Source: CAD feature listing. Evaluate the final solid. Frame: model axes, mm. A direction names the side the tool comes from. Round coordinates to 2 decimals unless told otherwise and drop trailing zeros. Loops run counter-clockwise (first coordinate to the right, second up) from the corner with the lowest first, then second, coordinate; pieces in that order, holes last. Notation, with made-up numbers: M -22,73 L -5,73 A26 cw -5,108 Z; hole C 1.5,-6 d11. An arc over 180 degrees is marked long. Write each question's results on one line, items separated by ' | '. Start each with the question number.
1. Section A-A on y = 47. Output: boundary loops of the cut face in (x, z), and give its area (3 significant figures).
2. Ray query, line 1 (Y direction, x = 1.3, z = 9); line 2 (X direction, y = 2.55, z = 59); line 3 (Y direction, x = 1.65, z = 64.25). Return the intervals inside material, ascending.
3. Set-up query: faces 1 (the flat face through (22, 4, 34)), 2 (the cylindrical face through (2.028, 20.808, 62.022)). Return all of +Z, -Z, +X, -X, +Y, -Y with unobstructed straight access to the full face (end or side cutting, diameter ignored); none if empty.
4. Section B-B on z = 9. Output: boundary loops of the cut face in (x, y).
5. Section D-D on y = 14. Output: boundary loops of the cut face in (x, z).
6. Section C-C on x = 11.5. Output: boundary loops of the cut face in (y, z), and give its area (3 significant figures).
7. Draft query along Y for faces 3 (the cylindrical face through (1.97, 50.07, 62.55)), 4 (the cylindrical face through (11.773, 1.972, 6.918)), 5 (the flat face through (2, 54, 34)). Return one class per face: released by +Y, released by -Y, zero draft, split by the parting line, or undercut.
8. Contact query for flat-ended pins moving along their axis: pin 1 Ø5 at (x, z) = (11.5, 9) entering from -Y; pin 2 Ø5.5 at (y, z) = (14, 3.75) entering from +X; pin 3 Ø1.2 at (y, z) = (20.5, 63) entering from +X; pin 4 Ø5 at (x, z) = (33, 27) entering from +Y. Output: stop coordinate, or through.
from build123d import *

# Parameters (mm, degrees)
BOSS_EXTRUDE1_DEPTH          = 68
M3_CLEARANCE_HOLE1_D         = 3.4
M3_CLEARANCE_HOLE1_DEPTH     = 5
M3_CLEARANCE_HOLE1_TIP       = 1.021463052
M5X0_8_TAPPED_HOLE1_D        = 4.2
M5X0_8_TAPPED_HOLE1_DEPTH    = 14
M5X0_8_TAPPED_HOLE1_TIP      = 1.2618073
FILLET1_R                    = 4
CHAMFER1_SIZE                = 0.5
M2_5X0_45_TAPPED_HOLE1_D     = 2.05
M2_5X0_45_TAPPED_HOLE1_DEPTH = 7.25
M2_5X0_45_TAPPED_HOLE1_TIP   = 0.615882135
M3X0_5_TAPPED_HOLE3_D        = 2.5
M3X0_5_TAPPED_HOLE3_DEPTH    = 8.5
M3X0_5_TAPPED_HOLE3_TIP      = 0.751075774


with BuildPart() as part:
    # Sketch1 → Boss-Extrude1 (new body)
    with BuildSketch(Plane.XY):
        Polygon((0, 0), (39, 0), (39, 4), (4, 4), (4, 54), (0, 54), align=None)
    extrude(amount=BOSS_EXTRUDE1_DEPTH)

    # M3 Clearance Hole1
    with Locations(Plane(origin=(4, 0, 0), x_dir=(0, 0, -1), z_dir=(1, 0, 0))):
        with Locations((-64.25, 50), (-3.75, 50), (-3.75, 14), (-64.25, 14)):
            Hole(M3_CLEARANCE_HOLE1_D / 2, depth=M3_CLEARANCE_HOLE1_DEPTH)
            with Locations((0, 0, -(M3_CLEARANCE_HOLE1_DEPTH + M3_CLEARANCE_HOLE1_TIP / 2))):  # 118° drill point
                Cone(0, M3_CLEARANCE_HOLE1_D / 2, M3_CLEARANCE_HOLE1_TIP, mode=Mode.SUBTRACT)

    # M5x0.8 Tapped Hole1
    with Locations(Plane(origin=(0, 4, 0), x_dir=(1, 0, 0), z_dir=(0, 1, 0))):
        with Locations((31.5, -59), (11.5, -59), (11.5, -9), (31.5, -9)):
            Hole(M5X0_8_TAPPED_HOLE1_D / 2, depth=M5X0_8_TAPPED_HOLE1_DEPTH)
            with Locations((0, 0, -(M5X0_8_TAPPED_HOLE1_DEPTH + M5X0_8_TAPPED_HOLE1_TIP / 2))):  # 118° drill point
                Cone(0, M5X0_8_TAPPED_HOLE1_D / 2, M5X0_8_TAPPED_HOLE1_TIP, mode=Mode.SUBTRACT)

    # Fillet1
    fillet1_edges = [part.edges().sort_by_distance(p)[0] for p in [
        (2, 54, 68),
        (2, 54, 0),
    ]]
    fillet(fillet1_edges, radius=FILLET1_R)

    # Chamfer1
    chamfer1_edges = [part.edges().sort_by_distance(p)[0] for p in [
        (0, 25, 68),
        (0, 25, 0),
        (0, 54, 34),
        (0, 52.828427125, 1.171572875),
        (0, 52.828427125, 66.828427125),
    ]]
    chamfer(chamfer1_edges, length=CHAMFER1_SIZE)

    # M2.5x0.45 Tapped Hole1
    with Locations(Plane.ZY):
        with Locations((5, 43.5), (63, 43.5), (63, 20.5), (5, 20.5)):
            Hole(M2_5X0_45_TAPPED_HOLE1_D / 2, depth=M2_5X0_45_TAPPED_HOLE1_DEPTH)
            with Locations((0, 0, -(M2_5X0_45_TAPPED_HOLE1_DEPTH + M2_5X0_45_TAPPED_HOLE1_TIP / 2))):  # 118° drill point
                Cone(0, M2_5X0_45_TAPPED_HOLE1_D / 2, M2_5X0_45_TAPPED_HOLE1_TIP, mode=Mode.SUBTRACT)

    # M3x0.5 Tapped Hole3
    with Locations(Plane.ZY):
        with Locations((9, 17), (9, 47), (59, 47), (59, 17)):
            Hole(M3X0_5_TAPPED_HOLE3_D / 2, depth=M3X0_5_TAPPED_HOLE3_DEPTH)
            with Locations((0, 0, -(M3X0_5_TAPPED_HOLE3_DEPTH + M3X0_5_TAPPED_HOLE3_TIP / 2))):  # 118° drill point
                Cone(0, M3X0_5_TAPPED_HOLE3_D / 2, M3X0_5_TAPPED_HOLE3_TIP, mode=Mode.SUBTRACT)


solid = part.part
Taken from the geometry:
1) outline: M 0,0.5 L 0.5,0 L 4,0 L 4,7.75 L 0,7.75 Z; M 0,10.25 L 4,10.25 L 4,57.75 L 0,57.75 Z; M 0,60.25 L 4,60.25 L 4,68 L 0.5,68 L 0,67.5 Z | area: 252 mm^2
2) line 1: 0 to 15.75, 18.25 to 45.75, 48.25 to 54 | line 2: 0 to 9.4, 13.6 to 29.4, 33.6 to 39 | line 3: 0 to 12.3, 15.7 to 48.3, 51.7 to 53.99
3) face 1: +Z, -Z, +X, +Y | face 2: +X, -X
4) outline: M 0,0 L 9.4,0 L 9.4,4 L 4,4 L 4,15.75 L 0,15.75 Z; M 0,18.25 L 4,18.25 L 4,45.75 L 0,45.75 Z; M 0,48.25 L 4,48.25 L 4,54 L 0.5,54 L 0,53.5 Z; M 13.6,0 L 29.4,0 L 29.4,4 L 13.6,4 Z; M 33.6,0 L 39,0 L 39,4 L 33.6,4 Z
5) outline: M 0,0.5 L 0.5,0 L 4,0 L 4,2.05 L 0,2.05 Z; M 0,5.45 L 4,5.45 L 4,62.55 L 0,62.55 Z; M 0,65.95 L 4,65.95 L 4,68 L 0.5,68 L 0,67.5 Z
6) outline: M 0,0 L 4,0 L 4,6.9 L 0,6.9 Z; M 0,11.1 L 4,11.1 L 4,56.9 L 0,56.9 Z; M 0,61.1 L 4,61.1 L 4,68 L 0,68 Z | area: 238 mm^2
7) face 3: undercut | face 4: zero draft | face 5: released by +Y
8) pin 1: y = 0 | pin 2: x = 4 | pin 3: through | pin 4: y = 4
